Verification items for this drawing (mm, ordinates from the low corner). Round coordinates to 2 decimals unless told otherwise and drop trailing zeros. Order: outer loops, then holes, each group sorted by start corner. A loop starts at its lowest first (then second) coordinate and runs counter-clockwise, first axis right, second up. Notation, with made-up numbers: M 16,35 L 50,35 A13 ccw 50,51 Z; hole C 70.5,47 d8. An arc over 180 degrees is marked long. Use CSV: the item, a comma, the result in double quotes. Start each with the question number.
Q1. Sectioned sample at C-C (z = 0.8). Enter the section's corners in (x, y), and give its area (3 significant figures).
Q2. Sectioned sample at B-B (x = 3). Enter the section's corners in (y, z), and give its area (3 significant figures).
Q3. Scan lines: line 1 (Y direction, x = 3, z = 0.85); line 2 (X direction, y = 3.25, z = 0.1); line 3 (X direction, y = 1, z = 0.35). Record each from-to range of solid material in increasing order.
Q4. Sectioned sample at A-A (y = 22). Enter the section's corners in (x, z), and give its area (3 significant figures).
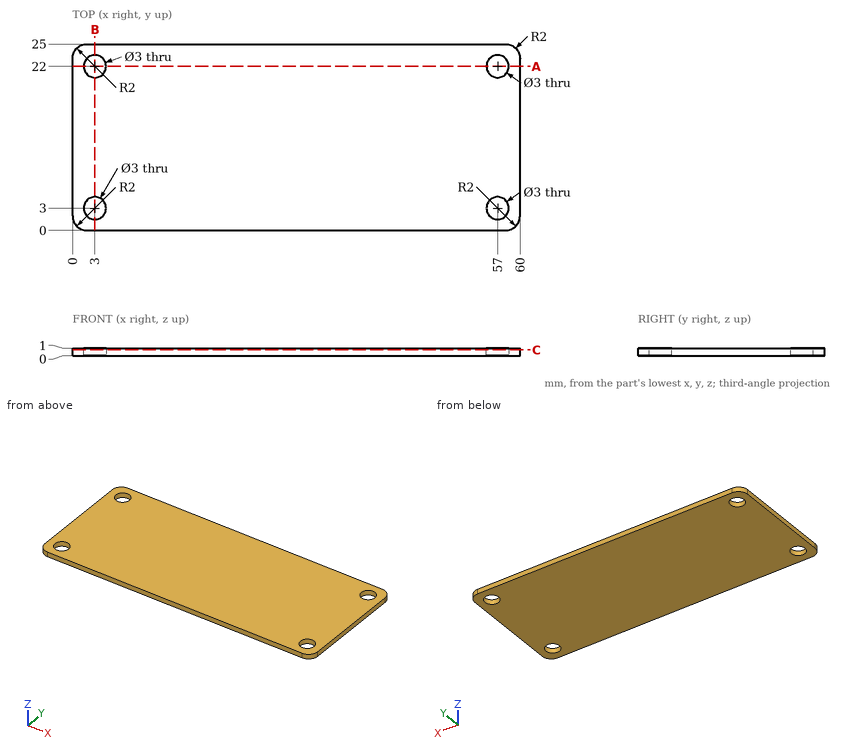
Verdict:
1,outline,"M 0,2 A2 ccw 2,0 L 58,0 A2 ccw 60,2 L 60,23 A2 ccw 58,25 L 2,25 A2 ccw 0,23 Z; hole C 3,3 d3; hole C 3,22 d3; hole C 57,3 d3; hole C 57,22 d3"
1,area,"1,470 mm²"
2,outline,"M 0,0 L 1.5,0 L 1.5,1 L 0,1 Z; M 4.5,0 L 20.5,0 L 20.5,1 L 4.5,1 Z; M 23.5,0 L 25,0 L 25,1 L 23.5,1 Z"
2,area,"19.0 mm²"
3,line 1,"y = 0 to 1.5, 4.5 to 20.5, 23.5 to 25"
3,line 2,"x = 0 to 1.52, 4.48 to 55.52, 58.48 to 60"
3,line 3,"x = 0.27 to 59.73"
4,outline,"M 0,0 L 1.5,0 L 1.5,1 L 0,1 Z; M 4.5,0 L 55.5,0 L 55.5,1 L 4.5,1 Z; M 58.5,0 L 60,0 L 60,1 L 58.5,1 Z"
4,area,"54.0 mm²"
